from build123d import *

# Parameters (mm, degrees)
EXTRUDE1_DEPTH = 0.3175


with BuildPart() as part:
    # Sketch1 → Extrude1 (new body, symmetric)
    with BuildSketch(Plane(origin=(0, 0, 0), x_dir=(0, 0, -1), z_dir=(1, 0, 0))):
        with BuildLine():
            ThreePointArc((-4.1021, 0), (0, -3.429), (4.1021, 0))
            ThreePointArc((4.1021, 0), (3.269449594, 1.105861316), (3.836428871, 2.368703526))
            ThreePointArc((3.836428871, 2.368703526), (4.032995284, 2.407207291), (4.192462169, 2.286))
            ThreePointArc((4.192462169, 2.286), (0, -4.7752), (-4.192462169, 2.286))
            ThreePointArc((-4.192462169, 2.286), (-4.032995284, 2.407207291), (-3.836428871, 2.368703526))
            ThreePointArc((-3.836428871, 2.368703526), (-3.269449594, 1.105861316), (-4.1021, 0))
        make_face()
    extrude(amount=EXTRUDE1_DEPTH, both=True)


solid = part.part
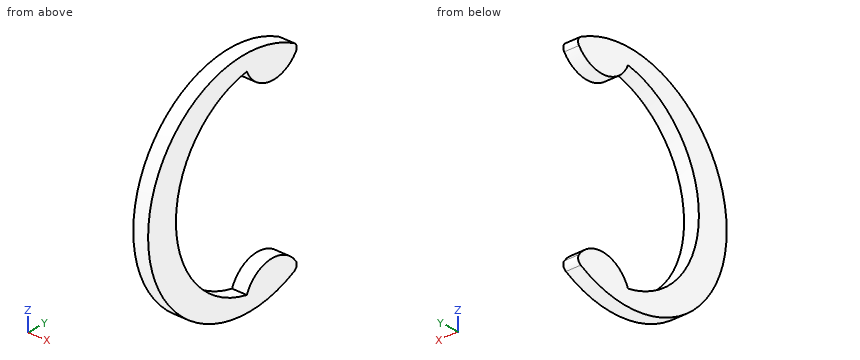
Check sheet for the modelled part. Datum: model origin and axes. Units: mm. Give positions to 0.01 mm unless a question says otherwise; leave off trailing zeros. Loops run counter-clockwise (first coordinate to the right, second up) from the corner with the lowest first, then second, coordinate; pieces in that order, holes last. Notation, with made-up numbers: M 32.25,4.25 L 40.25,4.25 A13 cw 40.25,19.25 Z; hole C 72.5,-21.75 d3. An arc over 180 degrees is marked long. Return JSON: item names as keys, results as strings. Group by question number.
1. Cross-section at A-A on y = 0.5. Record the boundary of the cut face in (x, z), plus the area to 3 significant figures.
2. Go/stop test with a flat-tipped pin: pin 1 (4 mm diameter, centred on y = -2.5, z = 2, fed in from +X). Record where the tip stops, or that it passes through.
3. Thickness scan on L1, parallel to Y at x = 0.15, z = 3.75; L2, parallel to Z at x = -0.1, y = 1.5; L3, parallel to Z at x = -0.2, y = -2.5. Record the ranges inside material, lowest first.
4. Cross-section at D-D on y = -0.75. Record the boundary of the cut face in (x, z).
5. Cross-section at B-B on x = 0. Record the boundary of the cut face in (y, z).
6. Cross-section at C-C on z = 3. Record the boundary of the cut face in (x, y), plus the area to 3 significant figures.
Return value:
{
 "1": {"outline": "M -0.32,-4.75 L 0.32,-4.75 L 0.32,-3.49 L -0.32,-3.49 Z; M -0.32,3.49 L 0.32,3.49 L 0.32,4.75 L -0.32,4.75 Z", "area": "1.60 mm^2"},
 "2": {"pin 1": "x = 0.32"},
 "3": {"L1": "-2.96 to -1.08, 0.21 to 2.3", "L2": "-4.53 to -3.28, 3.28 to 4.53", "L3": "-4.07 to -2.62, 2.62 to 4.07"},
 "4": {"outline": "M -0.32,-4.72 L 0.32,-4.72 L 0.32,-3.89 L -0.32,-3.89 Z; M -0.32,3.89 L 0.32,3.89 L 0.32,4.72 L -0.32,4.72 Z"},
 "5": {"outline": "M 0,-4.1 A4.17 cw 0,4.1 A1.36 ccw 2.37,3.84 A0.24 ccw 2.29,4.19 A4.78 ccw long 2.29,-4.19 A0.24 ccw 2.37,-3.84 A1.36 ccw Z"},
 "6": {"outline": "M -0.32,-3.72 L 0.32,-3.72 L 0.32,-2.15 L -0.32,-2.15 Z", "area": "0.991 mm^2"}
}
